Answer from the drawing. Dimensions are ordinates in mm from the lowest x, y and z of the part. Give positions to 0.01 mm unless a question says otherwise; leave off trailing zeros. Order: outer loops, then holes, each group sorted by start corner. A loop starts at its lowest first (then second) coordinate and runs counter-clockwise, first axis right, second up. Notation, with made-up numbers: (-20.75, 32) - (-14.75, 32) arc R12 ccw to (-14.75, 47) - close; hole circle Ø6 at (15.25, 12). An arc over 180 degrees is marked (long way). Use a Markdown table: item, result. Add a question column.
1) Find section B-B, the plane z = 34. Determine the outline of the cut face in (x, y).
2) Straight lines are drawn through the part: line 1 (Y direction, x = 12.7, z = 5.5) (3 decimals); line 2 (X direction, y = 393.7, z = 13.25) (3 decimals); line 3 (Y direction, x = 12.7, z = 11.5) (3 decimals). For each, find the intervals that lie inside material, in ascending order.
3) The mould has two halves that part along X. Classify the marked faces 1, 2 and 3: released by +X, released by -X, zero draft, split by the parting line, or undercut.
4) Find section A-A, the plane x = 22. Determine the outline of the cut face in (y, z), plus the area to 3 significant figures.
5) Flat-ended cylindrical pins translate along their axes: pin 1 (1.5 mm diameter, centred on x = 8, z = 13, fed in from +Y); pin 2 (10 mm diameter, centred on x = 14.5, z = 27.5, fed in from -Y); pin 3 (2 mm diameter, centred on x = 6.5, z = 13, fed in from -Y). Find the tip coordinate at first contact, or state that the pin passes through.
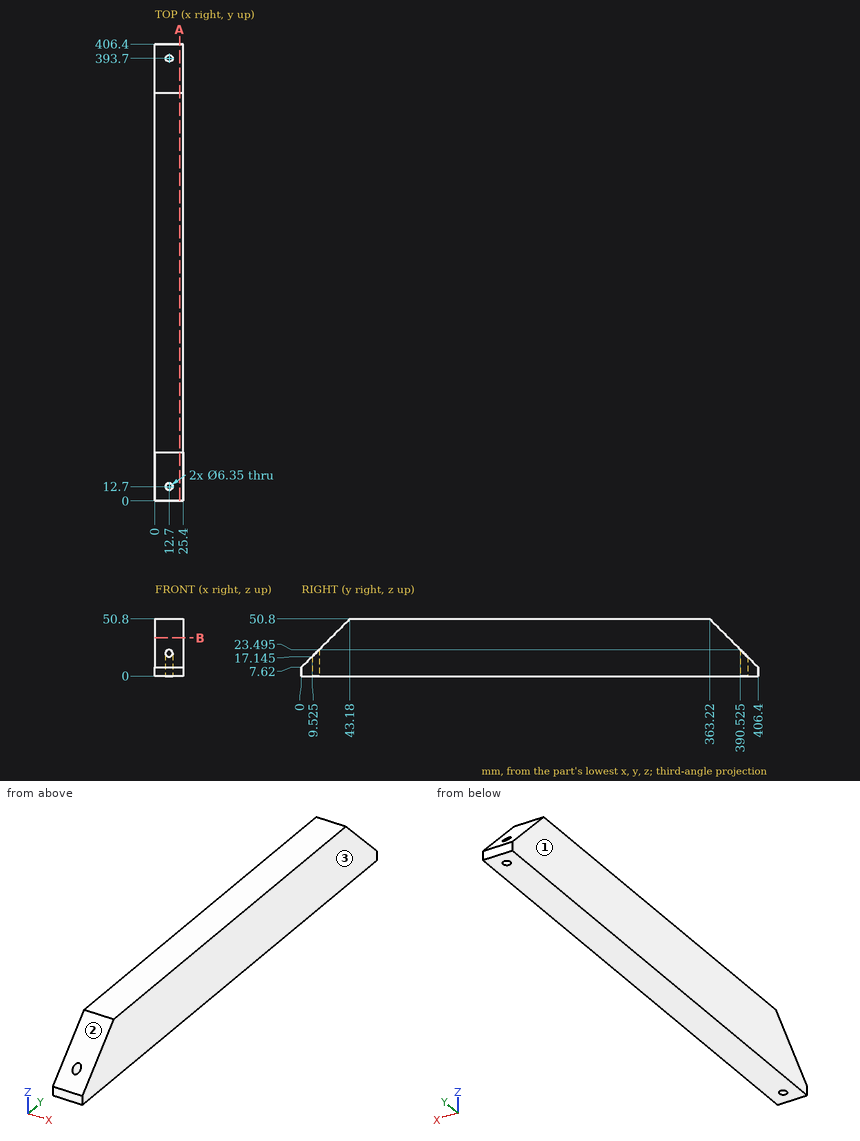
The answers:
| question | item | result |
|---|---|---|
| 1 | outline | (0, 26.38) - (25.4, 26.38) - (25.4, 380.02) - (0, 380.02) - close |
| 2 | line 1 | 0 to 9.525, 15.875 to 390.525, 396.875 to 406.4 |
| 2 | line 2 | 0 to 9.525, 15.875 to 25.4 |
| 2 | line 3 | 3.88 to 9.525, 15.875 to 390.525, 396.875 to 402.52 |
| 3 | face 1 | released by -X |
| 3 | face 2 | zero draft |
| 3 | face 3 | released by +X |
| 4 | outline | (0, 0) - (406.4, 0) - (406.4, 7.62) - (363.22, 50.8) - (43.18, 50.8) - (0, 7.62) - close |
| 4 | area | 18,800 mm2 |
| 5 | pin 1 | y = 401.77 |
| 5 | pin 2 | y = 14.9 |
| 5 | pin 3 | y = 4.38 |
